Geometry check sheet. Reference: the model listing, model coordinates, mm. Round coordinates to 2 decimals unless told otherwise and drop trailing zeros. Order: outer loops, then holes, each group sorted by start corner. A loop starts at its lowest first (then second) coordinate and runs counter-clockwise, first axis right, second up.
(1) Sectioned sample at A-A (z = 77). Record the boundary of the cut face in (x, y), plus the area to 3 significant figures.
(2) Sectioned sample at D-D (x = -7.5). Record the boundary of the cut face in (y, z).
(3) Material ranges on line 1 along Z through (x, y) = (-73.5, 9.25); line 2 along Z through (x, y) = (-82, 3.75); line 3 along X through (y, z) = (2.75, 58), recorded low to high.
(4) Sectioned sample at B-B (x = -73.5). Record the boundary of the cut face in (y, z).
(5) Go/stop test with flat-tipped pins: pin 1 (1.5 mm diameter, centred on y = 1.5, z = -49, fed in from -X); pin 2 (4 mm diameter, centred on x = -60, y = 7.5, fed in from +Z); pin 3 (3 mm diameter, centred on y = 2, z = 31, fed in from -X). Record where each tip stops, or that it passes through.
from build123d import *

# Parameters (mm, degrees)
SKETCH1_R           = 3.2
BOSS_EXTRUDE1_DEPTH = 10


with BuildPart() as part:
    # Sketch1 → Boss-Extrude1 (new body)
    with BuildSketch(Plane(origin=(0, 0, 0), x_dir=(1, 0, 0), z_dir=(0, 1, 0))):
        with BuildLine():
            Line((-47.977195104, 83.332534163), (-10.719183363, 46.074522422))
            ThreePointArc((-10.719183363, 46.074522422), (0, 50.514553548), (10.719183363, 46.074522422))
            Line((10.719183363, 46.074522422), (47.977195104, 83.332534163))
            ThreePointArc((47.977195104, 83.332534163), (83.332534163, 83.332534163), (83.332534163, 47.977195104))
            Line((83.332534163, 47.977195104), (46.074522422, 10.719183363))
            ThreePointArc((46.074522422, 10.719183363), (50.514553548, 0), (46.074522422, -10.719183363))
            Line((46.074522422, -10.719183363), (83.332534163, -47.977195104))
            ThreePointArc((83.332534163, -47.977195104), (83.332534163, -83.332534163), (47.977195104, -83.332534163))
            Line((47.977195104, -83.332534163), (10.719183363, -46.074522422))
            ThreePointArc((10.719183363, -46.074522422), (0, -50.514553548), (-10.719183363, -46.074522422))
            Line((-10.719183363, -46.074522422), (-47.977195104, -83.332534163))
            ThreePointArc((-47.977195104, -83.332534163), (-83.332534163, -83.332534163), (-83.332534163, -47.977195104))
            Line((-83.332534163, -47.977195104), (-46.074522422, -10.719183363))
            ThreePointArc((-46.074522422, -10.719183363), (-50.514553548, 0), (-46.074522422, 10.719183363))
            Line((-46.074522422, 10.719183363), (-83.332534163, 47.977195104))
            ThreePointArc((-83.332534163, 47.977195104), (-83.332534163, 83.332534163), (-47.977195104, 83.332534163))
        make_face()
        with Locations((-65.654864633, 65.654864633)):
            Circle(SKETCH1_R, mode=Mode.SUBTRACT)
        with Locations((65.654864633, -65.654864633)):
            Circle(SKETCH1_R, mode=Mode.SUBTRACT)
        with Locations((65.654864633, 65.654864633)):
            Circle(SKETCH1_R, mode=Mode.SUBTRACT)
        with Locations((-65.654864633, -65.654864633)):
            Circle(SKETCH1_R, mode=Mode.SUBTRACT)
    extrude(amount=BOSS_EXTRUDE1_DEPTH)


solid = part.part
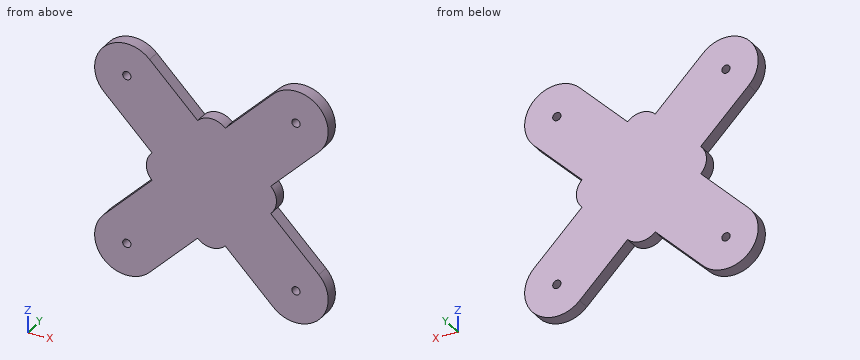
Answer below:
1. outline: (-87.93, 0) - (-41.64, 0) - (-41.64, 10) - (-87.93, 10) - close; (41.64, 0) - (87.93, 0) - (87.93, 10) - (41.64, 10) - close
1. area: 926 mm2
2. outline: (0, -48.53) - (10, -48.53) - (10, 48.53) - (0, 48.53) - close
3. line 1: z = -89.39 to -38.14, 38.14 to 89.39
3. line 2: z = -84.57 to -46.64, 46.64 to 84.57
3. line 3: x = -89.45 to -22.64, 22.64 to 89.45
4. outline: (0, -89.39) - (10, -89.39) - (10, -38.14) - (0, -38.14) - close; (0, 38.14) - (10, 38.14) - (10, 89.39) - (0, 89.39) - close
5. pin 1: stops at x = -84.94
5. pin 2: stops at z = 90.39
5. pin 3: stops at x = -67.86
